Work out the finished part from the listing and answer in its coordinate system (mm). Face numbers are marked on the shaded views. A direction names the side the tool comes from. Round coordinates to 2 decimals unless told otherwise and drop trailing zeros. Write each loop counter-clockwise with the first axis right and the second up, starting at its lowest first coordinate (ties: lowest second). Pieces come first, ordered by that corner, then holes.
1. Find section D-D (z = 13.75). Write down the section's boundary in (x, y).
2. Determine the mould class of the marked faces 4, 5 and 6 for opening direction Y: pulls with the +Y half, pulls with the -Y half, needs draft (parallel to the pull), parting line crosses it, or undercut.
3. A tool of negligible diameter and unlimited length cuts with its end or side. For the marked faces 1, 2 and 3, from which of +Z, -Z, +X, -X, +Y, -Y can it reach the whole face along a straight path? Write none if from no direction.
4. Find section A-A (x = 0). Write down the section's boundary in (y, z).
5. Find section B-B (y = -3.5). Write down the section's boundary in (x, z).
6. Straight lines are drawn through the part: probe 1 along Z at (x, y) = (0, -2.4); probe 2 along X at (y, z) = (-12.5, 4.5); probe 3 along Y at (x, z) = (-5.25, 18.75). For each, find the intervals that lie inside material, in ascending order.
7. Flat-ended cylindrical pins translate along their axes: pin 1 Ø1.9 at (x, z) = (-5.63, 13.75) entering from -Y; pin 2 Ø8.5 at (y, z) = (-15.5, 11) entering from -X; pin 3 Ø8 at (x, y) = (6.5, -15) entering from +Z; pin 4 Ø3.5 at (x, y) = (-6.5, -13.5) entering from +Z. Find the tip coordinate at first contact, or state that the pin passes through.
8. Find section C-C (z = 4). Write down the section's boundary in (x, y).
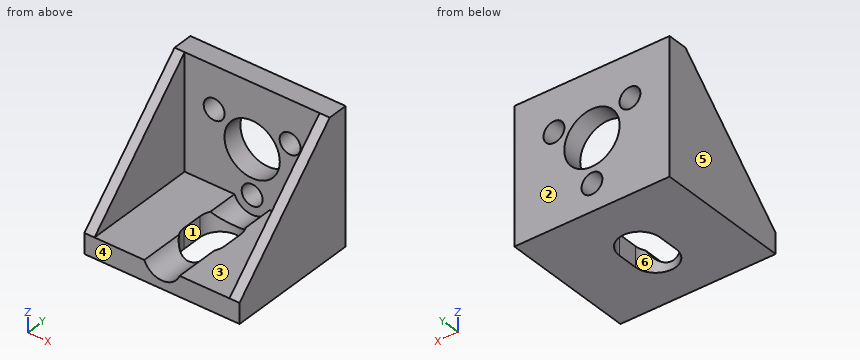
```python
from build123d import *

# Parameters (mm, degrees)
BOSS_EXTRUDE1_DEPTH   = 11.5
SKETCH2_W             = 17
SKETCH2_H             = 17
CUT_EXTRUDE1_DEPTH    = 10
CUT_EXTRUDE2_REACH    = 5
CORTE_EXTRUS_O1_REACH = 22
ESBO_O1_R             = 4.1
ESBO_O6_R             = 1.55
CORTE_EXTRUS_O5_DEPTH = 21
PADR_OCIRCULAR2_COUNT = 3
ESBO_O11_R            = 2.8
CORTE_EXTRUS_O8_DEPTH = 18.0000001


with BuildPart() as part:
    # Sketch1 → Boss-Extrude1 (new body, symmetric)
    with BuildSketch(Plane(origin=(0, 0, 0), x_dir=(0, 0, -1), z_dir=(1, 0, 0))):
        Polygon((0, 0), (-20, 0), (-20, -3), (-11.5, -11.5), (-3, -20), (0, -20), align=None)
    extrude(amount=BOSS_EXTRUDE1_DEPTH, both=True)

    # Sketch2 → Cut-Extrude1 (cut, symmetric)
    with BuildSketch(Plane(origin=(0, 0, 0), x_dir=(0, 0, -1), z_dir=(1, 0, 0))):
        with Locations((-11.5, -11.5)):
            Rectangle(SKETCH2_W, SKETCH2_H)
    extrude(amount=CUT_EXTRUDE1_DEPTH, both=True, mode=Mode.SUBTRACT)

    # Sketch3 → Cut-Extrude2 (cut, up to next)
    with BuildSketch(Plane.XY.offset(3), mode=Mode.PRIVATE) as cut_extrude2_sk1:
        with BuildLine():
            Line((-3, -9), (-3, -12))
            ThreePointArc((-3, -12), (0, -15), (3, -12))
            Line((3, -12), (3, -9))
            ThreePointArc((3, -9), (0, -6), (-3, -9))
        make_face()
    cut_extrude2_tool1 = extrude(cut_extrude2_sk1.sketch, amount=-CUT_EXTRUDE2_REACH, mode=Mode.PRIVATE) & part.part
    add(cut_extrude2_tool1.solids().sort_by_distance((0, -10.5, 3))[0], mode=Mode.SUBTRACT)

    # Esboço1 → Corte-extrusão1 (cut, up to next)
    with BuildSketch(Plane(origin=(0, 0, 0), x_dir=(1, 0, 0), z_dir=(0, 1, 0)), mode=Mode.PRIVATE) as corte_extrus_o1_sk1:
        with Locations((0, -10.5)):
            Circle(ESBO_O1_R)
    corte_extrus_o1_tool1 = extrude(corte_extrus_o1_sk1.sketch, amount=-CORTE_EXTRUS_O1_REACH, mode=Mode.PRIVATE) & part.part
    add(corte_extrus_o1_tool1.solids().sort_by_distance((0, 0, 10.5))[0], mode=Mode.SUBTRACT)

    # Esboço6 → Corte-extrusão5 (cut, through all)
    with BuildSketch(Plane(origin=(0, 0, 0), x_dir=(1, 0, 0), z_dir=(0, 1, 0))):
        with Locations((0, -4)):
            Circle(ESBO_O6_R)
    corte_extrus_o5 = extrude(amount=-CORTE_EXTRUS_O5_DEPTH, mode=Mode.SUBTRACT)

    # PadrãoCircular2: Corte-extrusão5 ×3 about axis
    padr_ocircular2_axis = Axis((0, 0, 10.5), (0, 1, 0))
    for i in range(1, PADR_OCIRCULAR2_COUNT):
        add(corte_extrus_o5.rotate(padr_ocircular2_axis, i * 360 / PADR_OCIRCULAR2_COUNT), mode=Mode.SUBTRACT)

    # Esboço11 → Corte-extrusão8 (cut, through all)
    with BuildSketch(Plane.XZ.offset(3)):
        with Locations((0, 4)):
            Circle(ESBO_O11_R)
    extrude(amount=CORTE_EXTRUS_O8_DEPTH, mode=Mode.SUBTRACT)


solid = part.part
```
Worked answers:
1. outline: (-11.5, -9.25) - (-10, -9.25) - (-10, -3) - (-7.18, -3) - (-7.18, 0) - (-11.5, 0) - close; (-4.08, -3) - (-2.5, -3) - (-2.5, 0) - (-4.08, 0) - close; (2.5, -3) - (4.08, -3) - (4.08, 0) - (2.5, 0) - close; (7.18, -3) - (10, -3) - (10, -9.25) - (11.5, -9.25) - (11.5, 0) - (7.18, 0) - close
2. face 4: pulls with the -Y half
2. face 5: needs draft
2. face 6: undercut
3. face 1: +Z, -Z
3. face 2: +Z, -Z, +X, -X, +Y
3. face 3: +Z, -Y
4. outline: (-20, 0) - (-15, 0) - (-15, 1.2) - (-20, 1.2) - close; (-6, 0) - (0, 0) - (0, 2.45) - (-3, 2.45) - (-3, 1.2) - (-6, 1.2) - close; (-3, 5.55) - (0, 5.55) - (0, 6.4) - (-3, 6.4) - close; (-3, 14.6) - (0, 14.6) - (0, 20) - (-3, 20) - close
5. outline: (-11.5, 0) - (11.5, 0) - (11.5, 19.5) - (10, 19.5) - (10, 3) - (2.62, 3) arc R2.8 cw to (-2.62, 3) - (-10, 3) - (-10, 19.5) - (-11.5, 19.5) - close
6. probe 1: z = 0 to 2.45, 5.55 to 6.4, 14.6 to 20
6. probe 2: x = -11.5 to -10, 10 to 11.5
6. probe 3: y = -3 to 0
7. pin 1: passes through
7. pin 2: stops at x = -11.5
7. pin 3: stops at z = 9.94
7. pin 4: stops at z = 3
8. outline: (-11.5, -19) - (-10, -19) - (-10, -3) - (-1.55, -3) - (-1.55, 0) - (-11.5, 0) - close; (1.55, -3) - (10, -3) - (10, -19) - (11.5, -19) - (11.5, 0) - (1.55, 0) - close
